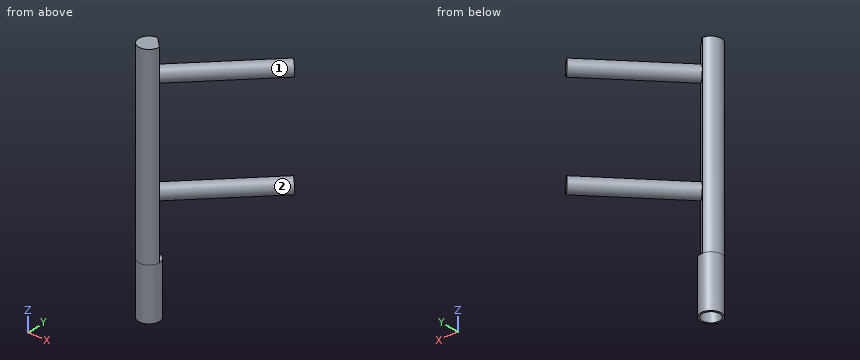
```python
from build123d import *

# Parameters (mm, degrees)
ESQUISSE1_R             = 3
BOSS_EXTRU_1_DEPTH      = 15
ESQUISSE2_R             = 2.5
ENL_V_MAT_EXTRU_1_DEPTH = 5
BOSS_EXTRU_2_DEPTH      = 55
ESQUISSE4_R             = 2.121320344
BOSS_EXTRU_3_DEPTH      = 30


with BuildPart() as part:
    # Esquisse1 → Boss.-Extru.1 (new body)
    with BuildSketch(Plane.XY):
        Circle(ESQUISSE1_R)
    extrude(amount=BOSS_EXTRU_1_DEPTH)

    # Esquisse2 → Enlèv. mat.-Extru.1 (cut)
    with BuildSketch(Plane(origin=(0, 0, 0), x_dir=(-1, 0, 0), z_dir=(0, 0, -1))):
        Circle(ESQUISSE2_R)
    extrude(amount=-ENL_V_MAT_EXTRU_1_DEPTH, mode=Mode.SUBTRACT)

    # Esquisse3 → Boss.-Extru.2 (add)
    with BuildSketch(Plane.XY.offset(15)):
        with BuildLine():
            Line((0, 3), (3, 0))
            ThreePointArc((3, 0), (-2.121320344, -2.121320344), (0, 3))
        make_face()
    extrude(amount=BOSS_EXTRU_2_DEPTH)

    # Esquisse4 → Boss.-Extru.3 (add)
    with BuildSketch(Plane(origin=(1.5, 1.5, 0), x_dir=(0, 0, -1), z_dir=(0.7071067811865477, 0.7071067811865475, 0))):
        with Locations(Location((-62, 0, 0), (0, 0, 90))):
            Circle(ESQUISSE4_R)
        with Locations(Location((-32, 0, 0), (0, 0, 90))):
            Circle(ESQUISSE4_R)
    extrude(amount=BOSS_EXTRU_3_DEPTH)


solid = part.part
```
Can you work these out from the model? Positions are in its coordinate system, mm. Face numbers are marked on the shaded views. Coordinates: 2 decimals unless noted, no trailing zeros. Order: outer loops, then holes, each group sorted by start corner. A loop starts at its lowest first (then second) coordinate and runs counter-clockwise, first axis right, second up. Notation, with made-up numbers: (-13.75, 81.5) - (35.25, 81.5) arc R22 cw to (35.25, 95.5) - close; hole circle Ø5 at (5.5, -14.5). An arc over 180 degrees is marked (long way). Answer in a Markdown table with one row per item.
1. For pin 1 (8 mm diameter, centred on y = 9, z = 31, fed in from -X); pin 2 (4 mm diameter, centred on x = 10.5, y = 12, fed in from -Z); pin 3 (12 mm diameter, centred on x = 6.5, y = 17, fed in from -Z), each with a flat end and sliding along its axis, tell me the tip position at first contact or that it passes through.
Reply:
| item | result |
|---|---|
| pin 1 | stops at x = 2.09 |
| pin 2 | stops at z = 29.88 |
| pin 3 | stops at z = 30.43 |
2. Suppose I cut it at A-A (z = 22.5). Please give me the cut outline in (x, y), and give its area (3 significant figures).
Reply:
| item | result |
|---|---|
| outline | (0, 3) arc R3 ccw (long way) to (3, 0) - close |
| area | 25.7 mm^2 |
3. If we mould it in two halves opening along Z, with no side actions, what happens to the marked faces 1 and 2? For each: pulls with the +Z half, pulls with the -Z half, needs draft (parallel to the pull), parting line crosses it, or undercut.
Reply:
| item | result |
|---|---|
| face 1 | undercut |
| face 2 | undercut |
4. If I drill on line 1 along Y through (x, z) = (0, 3.3); line 2 along Z through (x, y) = (4, 1.75); line 3 along Z through (x, y) = (17.5, 18.5), over which ranges is the centre line in solid material (lowest first)?
Reply:
| item | result |
|---|---|
| line 1 | y = -3 to -2.5, 2.5 to 3 |
| line 2 | z = 30.6 to 33.4, 60.6 to 63.4 |
| line 3 | z = 30 to 34, 60 to 64 |
